Could you check a few things on this model? Use its own coordinates, in mm. A direction names the side the tool comes from. Give positions to 0.01 mm unless a question says otherwise; leave off trailing zeros. Write each question's results on one line, items separated by ' | '. Start each with the question number.
from build123d import *

# Parameters (mm, degrees)
SKETCH2_W           = 920
SKETCH2_H           = 264
BOSS_EXTRUDE1_DEPTH = 10
SKETCH1_R           = 2.5
CUT_EXTRUDE2_DEPTH  = 18
SKETCH3_R           = 8
CUT_EXTRUDE3_DEPTH  = 6
SKETCH4_W           = 570
SKETCH4_H           = 264
CUT_EXTRUDE4_DEPTH  = 20
SKETCH7_R           = 3.4
SKETCH7_R_2         = 2.5
CUT_EXTRUDE5_DEPTH  = 20
SKETCH8_W           = 350
SKETCH8_H           = 5
CUT_EXTRUDE6_DEPTH  = 10
SKETCH9_R           = 1.25
SKETCH9_R_2         = 2
CUT_EXTRUDE7_DEPTH  = 10


with BuildPart() as part:
    # Sketch2 → Boss-Extrude1 (new body)
    with BuildSketch(Plane(origin=(0, 0, 0), x_dir=(1, 0, 0), z_dir=(0, 1, 0))):
        with Locations((460, 132)):
            Rectangle(SKETCH2_W, SKETCH2_H)
    extrude(amount=BOSS_EXTRUDE1_DEPTH)

    # Sketch1 → Cut-Extrude2 (cut)
    with BuildSketch(Plane(origin=(0, 10, 0), x_dir=(1, 0, 0), z_dir=(0, 1, 0))):
        with Locations(Location((40, 32, 0), (0, 0, 270))):
            Circle(SKETCH1_R)
        with Locations(Location((135, 32, 0), (0, 0, 270))):
            Circle(SKETCH1_R)
        with Locations(Location((230, 32, 0), (0, 0, 270))):
            Circle(SKETCH1_R)
        with Locations(Location((325, 32, 0), (0, 0, 270))):
            Circle(SKETCH1_R)
        with Locations(Location((420, 32, 0), (0, 0, 270))):
            Circle(SKETCH1_R)
        with Locations(Location((515, 32, 0), (0, 0, 270))):
            Circle(SKETCH1_R)
        with Locations(Location((610, 32, 0), (0, 0, 270))):
            Circle(SKETCH1_R)
        with Locations(Location((705, 32, 0), (0, 0, 270))):
            Circle(SKETCH1_R)
        with Locations(Location((800, 32, 0), (0, 0, 270))):
            Circle(SKETCH1_R)
        with Locations(Location((895, 32, 0), (0, 0, 270))):
            Circle(SKETCH1_R)
        with Locations(Location((135, 132, 0), (0, 0, 270))):
            Circle(SKETCH1_R)
        with Locations(Location((230, 132, 0), (0, 0, 270))):
            Circle(SKETCH1_R)
        with Locations(Location((325, 132, 0), (0, 0, 270))):
            Circle(SKETCH1_R)
        with Locations(Location((420, 132, 0), (0, 0, 270))):
            Circle(SKETCH1_R)
        with Locations(Location((515, 132, 0), (0, 0, 270))):
            Circle(SKETCH1_R)
        with Locations(Location((610, 132, 0), (0, 0, 270))):
            Circle(SKETCH1_R)
        with Locations(Location((705, 132, 0), (0, 0, 270))):
            Circle(SKETCH1_R)
        with Locations(Location((800, 132, 0), (0, 0, 270))):
            Circle(SKETCH1_R)
        with Locations(Location((895, 132, 0), (0, 0, 270))):
            Circle(SKETCH1_R)
        with Locations(Location((135, 232, 0), (0, 0, 270))):
            Circle(SKETCH1_R)
        with Locations(Location((230, 232, 0), (0, 0, 270))):
            Circle(SKETCH1_R)
        with Locations(Location((325, 232, 0), (0, 0, 270))):
            Circle(SKETCH1_R)
        with Locations(Location((420, 232, 0), (0, 0, 270))):
            Circle(SKETCH1_R)
        with Locations(Location((515, 232, 0), (0, 0, 270))):
            Circle(SKETCH1_R)
        with Locations(Location((610, 232, 0), (0, 0, 270))):
            Circle(SKETCH1_R)
        with Locations(Location((705, 232, 0), (0, 0, 270))):
            Circle(SKETCH1_R)
        with Locations(Location((800, 232, 0), (0, 0, 270))):
            Circle(SKETCH1_R)
        with Locations(Location((895, 232, 0), (0, 0, 270))):
            Circle(SKETCH1_R)
        with Locations(Location((40, 132, 0), (0, 0, 270))):
            Circle(SKETCH1_R)
        with Locations(Location((40, 232, 0), (0, 0, 270))):
            Circle(SKETCH1_R)
    extrude(amount=-CUT_EXTRUDE2_DEPTH, mode=Mode.SUBTRACT)

    # Sketch3 → Cut-Extrude3 (cut)
    with BuildSketch(Plane(origin=(0, 10, 0), x_dir=(1, 0, 0), z_dir=(0, 1, 0))):
        with Locations(Location((40, 32, 0), (0, 0, 270))):
            Circle(SKETCH3_R)
        with Locations(Location((135, 32, 0), (0, 0, 270))):
            Circle(SKETCH3_R)
        with Locations(Location((230, 32, 0), (0, 0, 270))):
            Circle(SKETCH3_R)
        with Locations(Location((325, 32, 0), (0, 0, 270))):
            Circle(SKETCH3_R)
        with Locations(Location((420, 32, 0), (0, 0, 270))):
            Circle(SKETCH3_R)
        with Locations(Location((515, 32, 0), (0, 0, 270))):
            Circle(SKETCH3_R)
        with Locations(Location((610, 32, 0), (0, 0, 270))):
            Circle(SKETCH3_R)
        with Locations(Location((705, 32, 0), (0, 0, 270))):
            Circle(SKETCH3_R)
        with Locations(Location((800, 32, 0), (0, 0, 270))):
            Circle(SKETCH3_R)
        with Locations(Location((895, 32, 0), (0, 0, 270))):
            Circle(SKETCH3_R)
        with Locations(Location((135, 132, 0), (0, 0, 270))):
            Circle(SKETCH3_R)
        with Locations(Location((230, 132, 0), (0, 0, 270))):
            Circle(SKETCH3_R)
        with Locations(Location((325, 132, 0), (0, 0, 270))):
            Circle(SKETCH3_R)
        with Locations(Location((420, 132, 0), (0, 0, 270))):
            Circle(SKETCH3_R)
        with Locations(Location((515, 132, 0), (0, 0, 270))):
            Circle(SKETCH3_R)
        with Locations(Location((610, 132, 0), (0, 0, 270))):
            Circle(SKETCH3_R)
        with Locations(Location((705, 132, 0), (0, 0, 270))):
            Circle(SKETCH3_R)
        with Locations(Location((800, 132, 0), (0, 0, 270))):
            Circle(SKETCH3_R)
        with Locations(Location((895, 132, 0), (0, 0, 270))):
            Circle(SKETCH3_R)
        with Locations(Location((135, 232, 0), (0, 0, 270))):
            Circle(SKETCH3_R)
        with Locations(Location((230, 232, 0), (0, 0, 270))):
            Circle(SKETCH3_R)
        with Locations(Location((325, 232, 0), (0, 0, 270))):
            Circle(SKETCH3_R)
        with Locations(Location((420, 232, 0), (0, 0, 270))):
            Circle(SKETCH3_R)
        with Locations(Location((515, 232, 0), (0, 0, 270))):
            Circle(SKETCH3_R)
        with Locations(Location((610, 232, 0), (0, 0, 270))):
            Circle(SKETCH3_R)
        with Locations(Location((705, 232, 0), (0, 0, 270))):
            Circle(SKETCH3_R)
        with Locations(Location((800, 232, 0), (0, 0, 270))):
            Circle(SKETCH3_R)
        with Locations(Location((895, 232, 0), (0, 0, 270))):
            Circle(SKETCH3_R)
        with Locations(Location((40, 132, 0), (0, 0, 270))):
            Circle(SKETCH3_R)
        with Locations(Location((40, 232, 0), (0, 0, 270))):
            Circle(SKETCH3_R)
    extrude(amount=-CUT_EXTRUDE3_DEPTH, mode=Mode.SUBTRACT)

    # Sketch4 → Cut-Extrude4 (cut)
    with BuildSketch(Plane(origin=(0, 10, 0), x_dir=(1, 0, 0), z_dir=(0, 1, 0))):
        with Locations((635, 132)):
            Rectangle(SKETCH4_W, SKETCH4_H)
    extrude(amount=-CUT_EXTRUDE4_DEPTH, mode=Mode.SUBTRACT)

    # Sketch7 → Cut-Extrude5 (cut)
    with BuildSketch(Plane(origin=(0, 10, 0), x_dir=(1, 0, 0), z_dir=(0, 1, 0))):
        with Locations(Location((10, 254, 0), (0, 0, 270))):
            Circle(SKETCH7_R)
        with Locations(Location((340, 254, 0), (0, 0, 270))):
            Circle(SKETCH7_R)
        with Locations(Location((340, 10, 0), (0, 0, 270))):
            Circle(SKETCH7_R)
        with Locations(Location((10, 10, 0), (0, 0, 270))):
            Circle(SKETCH7_R)
        with Locations(Location((10, 132, 0), (0, 0, 270))):
            Circle(SKETCH7_R_2)
        with Locations(Location((340, 132, 0), (0, 0, 270))):
            Circle(SKETCH7_R_2)
    extrude(amount=-CUT_EXTRUDE5_DEPTH, mode=Mode.SUBTRACT)

    # Sketch8 → Cut-Extrude6 (cut)
    with BuildSketch(Plane(origin=(0, 10, 0), x_dir=(1, 0, 0), z_dir=(0, 1, 0))):
        with Locations((175, 261.5)):
            Rectangle(SKETCH8_W, SKETCH8_H)
        with Locations((175, 2.5)):
            Rectangle(SKETCH8_W, SKETCH8_H)
    extrude(amount=-CUT_EXTRUDE6_DEPTH, mode=Mode.SUBTRACT)

    # Sketch9 → Cut-Extrude7 (cut)
    with BuildSketch(Plane(origin=(0, 10, 0), x_dir=(1, 0, 0), z_dir=(0, 1, 0))):
        with Locations(Location((10, 67.5, 0), (0, 0, 270))):
            Circle(SKETCH9_R)
        with Locations(Location((10, 42.5, 0), (0, 0, 270))):
            Circle(SKETCH9_R)
        with Locations(Location((304, 67.5, 0), (0, 0, 90))):
            Circle(SKETCH9_R)
        with Locations(Location((304, 42.5, 0), (0, 0, 90))):
            Circle(SKETCH9_R)
        with Locations(Location((73, 55, 0), (0, 0, 270))):
            Circle(SKETCH9_R)
        with Locations(Location((129, 55, 0), (0, 0, 270))):
            Circle(SKETCH9_R)
        with Locations(Location((185, 55, 0), (0, 0, 90))):
            Circle(SKETCH9_R)
        with Locations(Location((241, 55, 0), (0, 0, 90))):
            Circle(SKETCH9_R)
        with Locations(Location((10, 55, 0), (0, 0, 270))):
            Circle(SKETCH9_R_2)
        with Locations(Location((304, 55, 0), (0, 0, 90))):
            Circle(SKETCH9_R_2)
    extrude(amount=-CUT_EXTRUDE7_DEPTH, mode=Mode.SUBTRACT)


solid = part.part
1) I'm going to push flat-ended pins straight in: P1, Ø4.5, axis at x = 135, z = -32, coming from the +Y side; P2, Ø9.5, axis at x = 135, z = -32, coming from the +Y side. Where does each tip first touch, or does it pass through?
2) Please list where these lines run through material, in increasing order: line 1 (X direction, y = 7.3, z = -232); line 2 (X direction, y = 2.75, z = -254). Write a range as from..to.
3) Which directions (+Z, -Z, +X, -X, +Y, -Y) give clear straight access to the entire face, cutting with the end or side of a thin tool? Please do faces 4 (the face through (127.9, 7.04, -228.31)), 5 (the face through (173, 0, -134)).
4) Thinking about a two-plate mould opening in Z: for faces 1 (the face through (173, 5, -259)), 2 (the face through (173, 5, -5)), 3 (the face through (38, 4, -34)), which applies, pulls with the +Z half, pulls with the -Z half, needs draft (parallel to the pull), parting line crosses it, or undercut?
5) If we section it at A-A on y = 8: State how many separate pieces and enclosed holes the cut face has, plus the area to 3 significant figures.
Calculated:
1) P1: passes through | P2: stops at y = 4
2) line 1: x = 0..32, 48..127, 143..222, 238..317, 333..350 | line 2: x = 0..6.6, 13.4..336.6, 343.4..350
3) face 4: +Y | face 5: +Z, -Z, +X, -X, -Y
4) face 1: pulls with the -Z half | face 2: pulls with the +Z half | face 3: undercut
5) separate pieces: 1 | enclosed holes: 28 | area: 86,200 mm2
